Verification items for the finished model (mm, model axes). Coordinates: 2 decimals unless noted, no trailing zeros. Write each loop counter-clockwise with the first axis right and the second up, starting at its lowest first coordinate (ties: lowest second). Pieces come first, ordered by that corner, then holes. Notation, with made-up numbers: M 81,64.25 L 130,64.25 A14 ccw 130,78.25 Z; hole C 83,34.25 d5. An arc over 180 degrees is marked long. Answer in a Markdown table with one row per item.
Solid Edge part; units mm, degrees
sketch "Sketch1" plane through (0, 0, 0) normal (0, -1, 0) x (1, 0, 0)
  line L0 (8.5, 0) -> (8.5, 68.12)
  line L1 (-8.5, 68.12) -> (-8.5, 0)
  arc A0 (-8.5, 68.12) -> (8.5, 68.12) centre (0, 68.12) cw
  arc A1 (8.5, 0) -> (-8.5, 0) centre (0, 0) cw
extrude "Protrusion1" add sketch "Sketch1" against normal blind 1
sketch "Sketch2" plane through (0, 0, 0) normal (0, -1, 0) x (1, 0, 0)
  circle A0 centre (0, 68.12) radius 2.5
extrude "ExtrudedCutout_1" cut sketch "Sketch2" against normal blind 5
sketch "Sketch3" plane through (0, 0, 0) normal (0, -1, 0) x (1, 0, 0)
  circle A0 centre (0, 0) radius 2.5
extrude "ExtrudedCutout_2" cut sketch "Sketch3" against normal blind 5
1) Sectioned sample at D-D (z = 71.5). Record the cut outline in (x, y), then the cut area to 3 significant figures.
Response values:
| item | result |
|---|---|
| outline | M -7.8,0 L 7.8,0 L 7.8,1 L -7.8,1 Z |
| area | 15.6 mm² |
2) Sectioned sample at A-A (x = 0). Record the cut outline in (y, z).
Response values:
| item | result |
|---|---|
| outline | M 0,-8.5 L 1,-8.5 L 1,-2.5 L 0,-2.5 Z; M 0,2.5 L 1,2.5 L 1,65.62 L 0,65.62 Z; M 0,70.62 L 1,70.62 L 1,76.62 L 0,76.62 Z |
3) Thickness scan on L1, parallel to Z at x = 0, y = 0.6; L2, parallel to Z at x = 7, y = 0.25; L3, parallel to Z at x = -5.5, y = 0.75. Record the ranges inside material, lowest first. Write a range as [from, to].
Response values:
| item | result |
|---|---|
| L1 | z = [-8.5, -2.5], [2.5, 65.62], [70.62, 76.62] |
| L2 | z = [-4.82, 72.94] |
| L3 | z = [-6.48, 74.6] |
4) Release check for a two-part mould opening along X. For faces 1 (the face through (0, 0, 35)), 2 (the face through (-0.187, 0.493, -8.498)), 3 (the face through (-0.54, 0.49, 65.68)) record: +X half, -X half, draft (parallel to the pull), parting line (faces both ways), or undercut.
Response values:
| item | result |
|---|---|
| face 1 | draft |
| face 2 | parting line |
| face 3 | undercut |
5) Sectioned sample at C-C (x = -4). Record the cut outline in (y, z).
Response values:
| item | result |
|---|---|
| outline | M 0,-7.5 L 1,-7.5 L 1,75.62 L 0,75.62 Z |
6) Sectioned sample at B-B (y = 0.15). Record the cut outline in (x, z).
Response values:
| item | result |
|---|---|
| outline | M -8.5,0 A8.5 ccw 8.5,0 L 8.5,68.12 A8.5 ccw -8.5,68.12 Z; hole C 0,0 d5; hole C 0,68.12 d5 |
